Check sheet for the modelled part. Datum: model origin and axes. Units: mm. A direction names the side the tool comes from. Round coordinates to 2 decimals unless told otherwise and drop trailing zeros. Order: outer loops, then holes, each group sorted by start corner. A loop starts at its lowest first (then second) coordinate and runs counter-clockwise, first axis right, second up.
Autodesk Inventor part; units mm, degrees
ref_plane "BODY_TO_PARTS_XY" through (0, 17.5, 0) normal (0, 1, 0) x (1, 0, 0)
ref_plane "BODY_TO_PARTS_YZ" through (0, 17.5, 0) normal (1, 0, 0) x (0, 0, -1)
ref_plane "BODY_TO_PARTS_ZX" through (0, 17.5, 0) normal (0, 0, -1) x (0, 1, 0)
sketch "Sketch_1" plane through (0, 45.2, 0) normal (0, 1, 0) x (1, 0, 0)
  arc A0 (-1, 4.9) -> (-1, -4.9) centre (-1, 0) ccw
  line L0 (-1, -4.9) -> (1, -4.9)
  arc A1 (1, -4.9) -> (1, 4.9) centre (1, 0) ccw
  line L1 (1, 4.9) -> (-1, 4.9)
extrude "Extrusion1" add sketch "Sketch_1" against normal blind 1.2
sketch "Sketch_2" plane through (0, 0, 0) normal (0, 0, 1) x (1, 0, 0)
  line L0 (0, 41.1) -> (0, 44)
  line L1 (0, 44) -> (3.5, 44)
  line L2 (3.5, 44) -> (3.5, 43.1)
  line L3 (3.5, 43.1) -> (4.75, 43.1)
  line L4 (4.75, 43.1) -> (4.884, 42.6)
  line L5 (4.884, 42.6) -> (6, 41.9557)
  line L6 (6, 41.9557) -> (6, 41.1)
  line L7 (6, 41.1) -> (0, 41.1)
  line L8 (0, 41.1) -> (0, 44)
revolve "Revolution1" add sketch "Sketch_2" angle 360 about axis through (0, 41.1, 0) along (0, -1, 0)
sketch "Sketch_5" plane through (0, 0, 0) normal (0, 0, 1) x (1, 0, 0)
  line L0 (0, 24.6) -> (0, 41.1)
  line L1 (0, 41.1) -> (6.3865, 41.1)
  line L2 (6.3865, 41.1) -> (7, 40.4865)
  line L3 (7, 40.4865) -> (7, 25.2135)
  line L4 (7, 25.2135) -> (6.3865, 24.6)
  line L5 (6.3865, 24.6) -> (0, 24.6)
  line L6 (0, 24.6) -> (0, 41.1)
revolve "Revolution2" add sketch "Sketch_5" angle 360 about axis through (0, 24.6, 0) along (0, -1, 0)
thread "Thread1"
sketch "Sketch_6" plane through (0, 0, 0) normal (0, 0, 1) x (1, 0, 0)
  line L0 (0, 23.1) -> (0, 24.6)
  line L1 (0, 24.6) -> (6.5, 24.6)
  line L2 (6.5, 24.6) -> (6.5, 23.1)
  line L3 (6.5, 23.1) -> (0, 23.1)
  line L4 (0, 23.1) -> (0, 24.6)
revolve "Revolution3" add sketch "Sketch_6" angle 360 about axis through (0, 23.1, 0) along (0, -1, 0)
sketch "Sketch_8" plane through (0, 0, 0) normal (0, 0, 1) x (1, 0, 0)
  line L0 (0, 17.5) -> (0, 23.1)
  line L1 (0, 23.1) -> (6, 23.1)
  line L2 (6, 23.1) -> (8.4, 22.4569)
  line L3 (8.4, 22.4569) -> (8.4, 18.1431)
  line L4 (8.4, 18.1431) -> (6, 17.5)
  line L5 (6, 17.5) -> (0, 17.5)
  line L6 (0, 17.5) -> (0, 23.1)
revolve "Revolution4" add sketch "Sketch_8" angle 360 about axis through (0, 17.5, 0) along (0, -1, 0)
sketch "Sketch_9" plane through (0, 23.1, 0) normal (0, 1, 0) x (1, 0, 0)
  line L0 (-12, -12) -> (12, -12)
  line L1 (12, -12) -> (12, 12)
  line L2 (12, 12) -> (-12, 12)
  line L3 (-12, 12) -> (-12, -12)
  line L4 (-8.0829, 0) -> (-4.0415, -7)
  line L5 (-4.0415, -7) -> (4.0415, -7)
  line L6 (4.0415, -7) -> (8.0829, 0)
  line L7 (8.0829, 0) -> (4.0415, 7)
  line L8 (4.0415, 7) -> (-4.0415, 7)
  line L9 (-4.0415, 7) -> (-8.0829, 0)
extrude "Extrusion2" cut sketch "Sketch_9" against normal blind 5.6
sketch "Sketch_10" plane through (0, 0, 0) normal (0, 0, 1) x (1, 0, 0)
  line L0 (0, 17.5) -> (0, 19.1)
  line L1 (0, 19.1) -> (11, 19.1)
  line L2 (11, 19.1) -> (11, 17.5)
  line L3 (11, 17.5) -> (0, 17.5)
  line L4 (0, 17.5) -> (0, 19.1)
revolve "Revolution5" add sketch "Sketch_10" angle 360 about axis through (0, 17.5, 0) along (0, -1, 0)
sketch "Sketch_12" plane through (0, 0, 0) normal (0, 0, 1) x (1, 0, 0)
  line L0 (0, 33.5) -> (0, 45.2)
  line L1 (0, 45.2) -> (3, 45.2)
  line L2 (3, 45.2) -> (3, 33.5)
  line L3 (3, 33.5) -> (0, 33.5)
  line L4 (0, 33.5) -> (0, 45.2)
revolve "Revolution6" cut sketch "Sketch_12" angle 360 about axis through (0, 33.5, 0) along (0, -1, 0)
sketch "Sketch_22" plane through (0, 0, 0) normal (0, 0, 1) x (1, 0, 0)
  line L0 (0, 17.5) -> (0, 0)
  line L1 (0, 0) -> (-19.5554, 0)
  line L2 (-19.5554, 0) -> (-20, 0.77)
  line L3 (-20, 0.77) -> (-16.3829, 2.5689)
  arc A0 (-16.3829, 2.5689) -> (-12.5, 8.8366) centre (-19.5, 8.8366) ccw
  line L4 (-12.5, 8.8366) -> (-12.5, 14.5)
  arc A1 (-9.5, 17.5) -> (-12.5, 14.5) centre (-9.5, 14.5) ccw
  line L5 (-9.5, 17.5) -> (0, 17.5)
  line L6 (0, 17.5) -> (0, 0)
revolve "Revolution7" add sketch "Sketch_22" angle 360 about axis through (0, 17.5, 0) along (0, 1, 0)
ref_plane "BODY_TO_PARTS_XY" through (0, 17.5, 0) normal (0, 1, 0) x (1, 0, 0)
ref_plane "BODY_TO_PARTS_YZ" through (0, 17.5, 0) normal (1, 0, 0) x (0, 0, -1)
ref_plane "BODY_TO_PARTS_ZX" through (0, 17.5, 0) normal (0, 0, -1) x (0, 1, 0)
ref_plane "body_to_nut1_XY" through (0, 30.3, 0) normal (0, 1, 0) x (1, 0, 0)
ref_plane "body_to_nut1_YZ" through (0, 30.3, 0) normal (1, 0, 0) x (0, 0, -1)
ref_plane "body_to_nut1_ZX" through (0, 30.3, 0) normal (0, 0, -1) x (0, 1, 0)
ref_plane "body_to_nut2_XY" through (0, 24.7, 0) normal (0, 1, 0) x (1, 0, 0)
ref_plane "body_to_nut2_YZ" through (0, 24.7, 0) normal (1, 0, 0) x (0, 0, -1)
ref_plane "body_to_nut2_ZX" through (0, 24.7, 0) normal (0, 0, -1) x (0, 1, 0)
ref_plane "body_to_nut3_XY" through (0, 34.6, 0) normal (0, 1, 0) x (1, 0, 0)
ref_plane "body_to_nut3_YZ" through (0, 34.6, 0) normal (1, 0, 0) x (0, 0, -1)
ref_plane "body_to_nut3_ZX" through (0, 34.6, 0) normal (0, 0, -1) x (0, 1, 0)
ref_plane "body_to_nut4_XY" through (0, 27.6, 0) normal (0, 1, 0) x (1, 0, 0)
ref_plane "body_to_nut4_YZ" through (0, 27.6, 0) normal (1, 0, 0) x (0, 0, -1)
ref_plane "body_to_nut4_ZX" through (0, 27.6, 0) normal (0, 0, -1) x (0, 1, 0)
ref_plane "作業平面17" through (0, 0, 10) normal (0, 0, 1) x (1, 0, 0)
sketch "スケッチ11" plane through (0, 0, 10) normal (0, 0, 1) x (1, 0, 0)
  arc A0 (-16.3829, 2.5689) -> (-12.5, 8.8366) centre (-19.5, 8.8366) ccw
  line L0 (0, 0) -> (-19.5554, 0)
  line L1 (-19.5554, 0) -> (-20, 0.77)
  line L2 (-5.9, 44) -> (-1, 44)
  line L3 (-1, 45.2) -> (-5.9, 45.2)
  line L4 (-1, 45.2) -> (-1, 44)
  line L5 (-4.884, 42.6) -> (4.884, 42.6)
  line L6 (-4.884, 42.6) -> (4.884, 42.6)
  line L7 (-4.75, 43.1) -> (4.75, 43.1)
  line L8 (-3.5, 43.1) -> (3.5, 43.1)
  line L9 (-4.75, 43.1) -> (4.75, 43.1)
  line L10 (-1, 44) -> (1, 44)
  line L11 (1, 44) -> (-1, 44)
  line L12 (3.5, 44) -> (-3.5, 44)
  line L13 (-3.5, 43.1) -> (3.5, 43.1)
  line L14 (3.5, 44) -> (-3.5, 44)
  line L15 (1, 44) -> (5.9, 44)
  line L16 (3.5, 44) -> (-3.5, 44)
  line L17 (-1, 44) -> (-1, 44)
  line L18 (-1, 44) -> (1, 44)
  line L19 (1, 44) -> (1, 44)
  line L20 (1, 44) -> (-1, 44)
  line L21 (-3, 45.2) -> (3, 45.2)
  line L22 (-1, 45.2) -> (-1, 45.2)
  line L23 (-1, 45.2) -> (1, 45.2)
  line L24 (1, 45.2) -> (1, 45.2)
  line L25 (1, 45.2) -> (-1, 45.2)
  line L26 (5.9, 45.2) -> (1, 45.2)
  line L27 (1, 45.2) -> (1, 45.2)
  line L28 (1, 45.2) -> (1, 44)
  line L29 (1, 44) -> (1, 44)
  line L30 (1, 45.2) -> (1, 44)
  line L31 (1, 45.2) -> (1, 44)
  line L32 (-1, 45.2) -> (1, 45.2)
  line L33 (-1, 45.2) -> (1, 45.2)
  line L34 (-1, 45.2) -> (-1, 44)
  line L35 (1, 44) -> (-1, 44)
  line L36 (1, 45.2) -> (1, 44)
  line L37 (1, 45.2) -> (-1, 45.2)
  line L38 (1, 45.2) -> (1, 44)
  line L39 (1, 45.2) -> (-1, 45.2)
  line L40 (1, 45.2) -> (1, 44)
  line L41 (-1, 44) -> (1, 44)
  line L42 (-1, 45.2) -> (-1, 44)
  line L43 (-3, 45.2) -> (3, 45.2)
  line L44 (-4.75, 43.1) -> (4.75, 43.1)
  line L45 (-3.5, 43.1) -> (3.5, 43.1)
  line L46 (-3, 33.5) -> (3, 33.5)
  line L47 (-3, 45.2) -> (3, 45.2)
  line L48 (-6, 41.9557) -> (6, 41.9557)
  line L49 (-4.884, 42.6) -> (4.884, 42.6)
  line L50 (-6, 41.9557) -> (6, 41.9557)
  line L51 (-6, 41.1) -> (6, 41.1)
  line L52 (-6, 41.9557) -> (6, 41.9557)
  line L53 (-6, 41.1) -> (6, 41.1)
  line L54 (-3, 33.5) -> (3, 33.5)
  line L55 (-3, 33.5) -> (3, 33.5)
  line L56 (-6.3865, 41.1) -> (6.3865, 41.1)
  line L57 (-6.3865, 41.1) -> (6.3865, 41.1)
  line L58 (-6, 41.1) -> (6, 41.1)
  line L59 (-7, 40.4865) -> (7, 40.4865)
  line L60 (-7, 25.2135) -> (7, 25.2135)
  line L61 (-7, 40.4865) -> (7, 40.4865)
  line L62 (-7, 40.4865) -> (7, 40.4865)
  line L63 (-6.3865, 41.1) -> (6.3865, 41.1)
  line L64 (-7, 25.2135) -> (7, 25.2135)
  line L65 (-6.5, 23.1) -> (6.5, 23.1)
  line L66 (-6.3865, 24.6) -> (6.3865, 24.6)
  line L67 (-6.5, 24.6) -> (6.5, 24.6)
  line L68 (6, 23.1) -> (-6, 23.1)
  line L69 (-8.0829, 22.5419) -> (-8.0829, 19.1)
  line L70 (-4.0415, 22.5419) -> (-4.0415, 19.1)
  line L71 (4.0415, 22.5419) -> (4.0415, 19.1)
  line L72 (8.0829, 22.5419) -> (8.0829, 19.1)
  line L73 (-4.0415, 22.5419) -> (-4.0415, 19.1)
  line L74 (4.0415, 22.5419) -> (4.0415, 19.1)
  line L75 (4.0415, 19.1) -> (-4.0415, 19.1)
  line L76 (4.0415, 19.1) -> (-4.0415, 19.1)
  line L77 (-4.0415, 22.5419) -> (-4.0415, 19.1)
  line L78 (4.0415, 22.5419) -> (4.0415, 19.1)
  line L79 (-6.5, 24.6) -> (6.5, 24.6)
  line L80 (-6.3865, 24.6) -> (6.3865, 24.6)
  line L81 (-6.3865, 24.6) -> (6.3865, 24.6)
  line L82 (-7, 25.2135) -> (7, 25.2135)
  line L83 (-6.5, 23.1) -> (6.5, 23.1)
  line L84 (-6.5, 24.6) -> (6.5, 24.6)
  line L85 (-4.0415, 19.1) -> (-8.0829, 19.1)
  line L86 (8.0829, 19.1) -> (4.0415, 19.1)
  line L87 (8.0829, 19.1) -> (4.0415, 19.1)
  line L88 (4.0415, 22.5419) -> (4.0415, 19.1)
  line L89 (8.0829, 22.5419) -> (8.0829, 19.1)
  line L90 (-4.0415, 19.1) -> (-8.0829, 19.1)
  line L91 (-8.0829, 22.5419) -> (-8.0829, 19.1)
  line L92 (-4.0415, 22.5419) -> (-4.0415, 19.1)
  line L93 (-8.0829, 19.1) -> (-4.0415, 19.1)
  line L94 (-8.0829, 19.1) -> (-4.0415, 19.1)
  line L95 (-4.0415, 22.5419) -> (-4.0415, 19.1)
  line L96 (-8.0829, 22.5419) -> (-8.0829, 19.1)
  line L97 (6, 23.1) -> (-6, 23.1)
  line L98 (-4.0415, 19.1) -> (4.0415, 19.1)
  line L99 (-4.0415, 19.1) -> (4.0415, 19.1)
  line L100 (4.0415, 22.5419) -> (4.0415, 19.1)
  line L101 (-4.0415, 22.5419) -> (-4.0415, 19.1)
  line L102 (6, 23.1) -> (-6, 23.1)
  line L103 (-6.5, 23.1) -> (6.5, 23.1)
  line L104 (4.0415, 19.1) -> (8.0829, 19.1)
  line L105 (4.0415, 19.1) -> (8.0829, 19.1)
  line L106 (8.0829, 22.5419) -> (8.0829, 19.1)
  line L107 (4.0415, 22.5419) -> (4.0415, 19.1)
  line L108 (-1, 45.2) -> (-1, 44)
  line L109 (-1, 45.2) -> (-1, 45.2)
  line L110 (-1, 45.2) -> (-1, 44)
  line L111 (-1, 44) -> (-1, 44)
  line L112 (-1, 45.2) -> (-1, 44)
  line L113 (-11, 19.1) -> (11, 19.1)
  line L114 (-11, 17.5) -> (11, 17.5)
  line L115 (-9.5, 17.5) -> (9.5, 17.5)
  line L116 (12.5, 14.5) -> (-12.5, 14.5)
  line L117 (12.5, 8.8366) -> (-12.5, 8.8366)
  line L118 (-11, 19.1) -> (11, 19.1)
  line L119 (4.0415, 19.1) -> (-4.0415, 19.1)
  line L120 (8.0829, 19.1) -> (4.0415, 19.1)
  line L121 (4.0415, 19.1) -> (8.0829, 19.1)
  line L122 (-4.0415, 19.1) -> (4.0415, 19.1)
  line L123 (-8.0829, 19.1) -> (-4.0415, 19.1)
  line L124 (-4.0415, 19.1) -> (-8.0829, 19.1)
  line L125 (-11, 17.5) -> (11, 17.5)
  line L126 (-11, 19.1) -> (11, 19.1)
  line L127 (-9.5, 17.5) -> (9.5, 17.5)
  line L128 (12.5, 14.5) -> (-12.5, 14.5)
  line L129 (12.5, 14.5) -> (-12.5, 14.5)
  line L130 (12.5, 8.8366) -> (-12.5, 8.8366)
  line L131 (-11, 17.5) -> (11, 17.5)
  line L132 (-9.5, 17.5) -> (9.5, 17.5)
  line L133 (0, 17.5) -> (0, 19.1)
  line L134 (0, 19.1) -> (11, 19.1)
  line L135 (11, 19.1) -> (11, 17.5)
  line L136 (11, 17.5) -> (0, 17.5)
  line L137 (0, 17.5) -> (0, 19.1)
  line L138 (0, 33.5) -> (0, 45.2)
  line L139 (0, 45.2) -> (3, 45.2)
  line L140 (3, 45.2) -> (3, 33.5)
  line L141 (3, 33.5) -> (0, 33.5)
  line L142 (0, 33.5) -> (0, 45.2)
  line L143 (0, 17.5) -> (0, 0)
  line L144 (-20, 0.77) -> (-16.3829, 2.5689)
  line L145 (-12.5, 8.8366) -> (-12.5, 14.5)
  arc A1 (-9.5, 17.5) -> (-12.5, 14.5) centre (-9.5, 14.5) ccw
  line L146 (-9.5, 17.5) -> (0, 17.5)
  line L147 (0, 17.5) -> (0, 0)
  line L148 (0, 17.5) -> (0, 23.1)
  line L149 (0, 23.1) -> (6, 23.1)
  line L150 (6, 23.1) -> (8.4, 22.4569)
  line L151 (8.4, 22.4569) -> (8.4, 18.1431)
  line L152 (8.4, 18.1431) -> (6, 17.5)
  line L153 (6, 17.5) -> (0, 17.5)
  line L154 (0, 17.5) -> (0, 23.1)
  line L155 (0, 23.1) -> (0, 24.6)
  line L156 (0, 24.6) -> (6.5, 24.6)
  line L157 (6.5, 24.6) -> (6.5, 23.1)
  line L158 (6.5, 23.1) -> (0, 23.1)
  line L159 (0, 23.1) -> (0, 24.6)
  line L160 (0, 24.6) -> (0, 41.1)
  line L161 (0, 41.1) -> (6.3865, 41.1)
  line L162 (6.3865, 41.1) -> (7, 40.4865)
  line L163 (7, 40.4865) -> (7, 25.2135)
  line L164 (7, 25.2135) -> (6.3865, 24.6)
  line L165 (6.3865, 24.6) -> (0, 24.6)
  line L166 (0, 24.6) -> (0, 41.1)
  line L167 (0, 41.1) -> (0, 44)
  line L168 (0, 44) -> (3.5, 44)
  line L169 (3.5, 44) -> (3.5, 43.1)
  line L170 (3.5, 43.1) -> (4.75, 43.1)
  line L171 (4.75, 43.1) -> (4.884, 42.6)
  line L172 (4.884, 42.6) -> (6, 41.9557)
  line L173 (6, 41.9557) -> (6, 41.1)
  line L174 (6, 41.1) -> (0, 41.1)
  line L175 (0, 41.1) -> (0, 44)
properties part number "MVFKN40-1-1"
1) Sectioned sample at A-A on y = 18.5. Record the cut outline in (x, z), and give its area (3 significant figures).
2) Scan lines: line 1 (Z direction, x = 0, y = 36.25); line 2 (Z direction, x = 0, y = 41.75); line 3 (X direction, y = 35, z = 2). Record each from-to range of solid material in increasing order.
3) Set-up check for faces 5 (the face through (-5.9, 44.6, -0.1)), 6 (the face through (6.034, 20.992, 3.549)), 7 (the face through (0, 21, 7)), 8 (the face through (-4, 43.1, 0)), 9 (the face through (-2.38, 18.29, -10.74)): record each of +Z, -Z, +X, -X, +Y, -Y from which the full face is reachable in a straight line by a thin tool's end or side.
4) Gauge pin test, flat ends, axial feed: pin 1 (7.5 mm diameter, centred on x = -0.5, z = -0.5, fed in from +Y); pin 2 (10 mm diameter, centred on x = 3, y = 8.5, fed in from +Z); pin 3 (0.6 mm diameter, centred on x = 0, y = 44.5, fed in from +Z); pin 4 (12 mm diameter, centred on y = 28.5, z = 1, fed in from -X). Record the tip position at first contact, or that the pin passes through.
5) Draft check along Y on faces 1 (the face through (-5.158, 23.84, -3.955)), 2 (the face through (0, 33.5, 0)), 3 (the face through (6.09, 20.99, -3.45)), 4 (the face through (3.233, 43.544, -1.341)). Enter one of: pulls with the +Y half, pulls with the -Y half, needs draft (parallel to the pull), parting line crosses it, or undercut.
Values found:
1. outline: circle Ø22 at (0, 0)
1. area: 380 mm2
2. line 1: z = -7 to -3, 3 to 7
2. line 2: z = -6 to -3, 3 to 6
2. line 3: x = -6.71 to -2.24, 2.24 to 6.71
3. face 5: -X, +Y
3. face 6: +Z, +X, +Y
3. face 7: +Z, +X, -X, +Y
3. face 8: none
3. face 9: +Y
4. pin 1: stops at y = 45.2
4. pin 2: stops at z = 14.73
4. pin 3: stops at z = 4.9
4. pin 4: stops at x = -8
5. face 1: undercut
5. face 2: pulls with the +Y half
5. face 3: needs draft
5. face 4: undercut
